Geometry check sheet. Reference: drawing and pictorial views, mm from the part's lowest x, y, z. Round coordinates to 2 decimals unless told otherwise and drop trailing zeros. Order: outer loops, then holes, each group sorted by start corner. A loop starts at its lowest first (then second) coordinate and runs counter-clockwise, first axis right, second up.
(1) Cross-section at B-B on z = 76.5. Enter the section's corners in (x, y), and give its area (3 significant figures).
(2) Cross-section at A-A on x = 61. Enter the section's corners in (y, z), and give its area (3 significant figures).
(3) Gauge pin test, flat ends, axial feed: P1, Ø1.4, axis at x = 37.5, y = 2, coming from the +Z side; P2, Ø1.5, axis at y = 1, z = 104.5, coming from the -X side (3 decimals); P3, Ø1.4, axis at x = 33, y = 1.5, coming from the -Z side. Record the tip position at first contact, or that the pin passes through.
(4) Thickness scan on L1, parallel to Z at x = 32.5, y = 2.15; L2, parallel to X at y = 0.2, z = 99; L3, parallel to Z at x = 62, y = 0.35. Record the ranges inside material, lowest first.
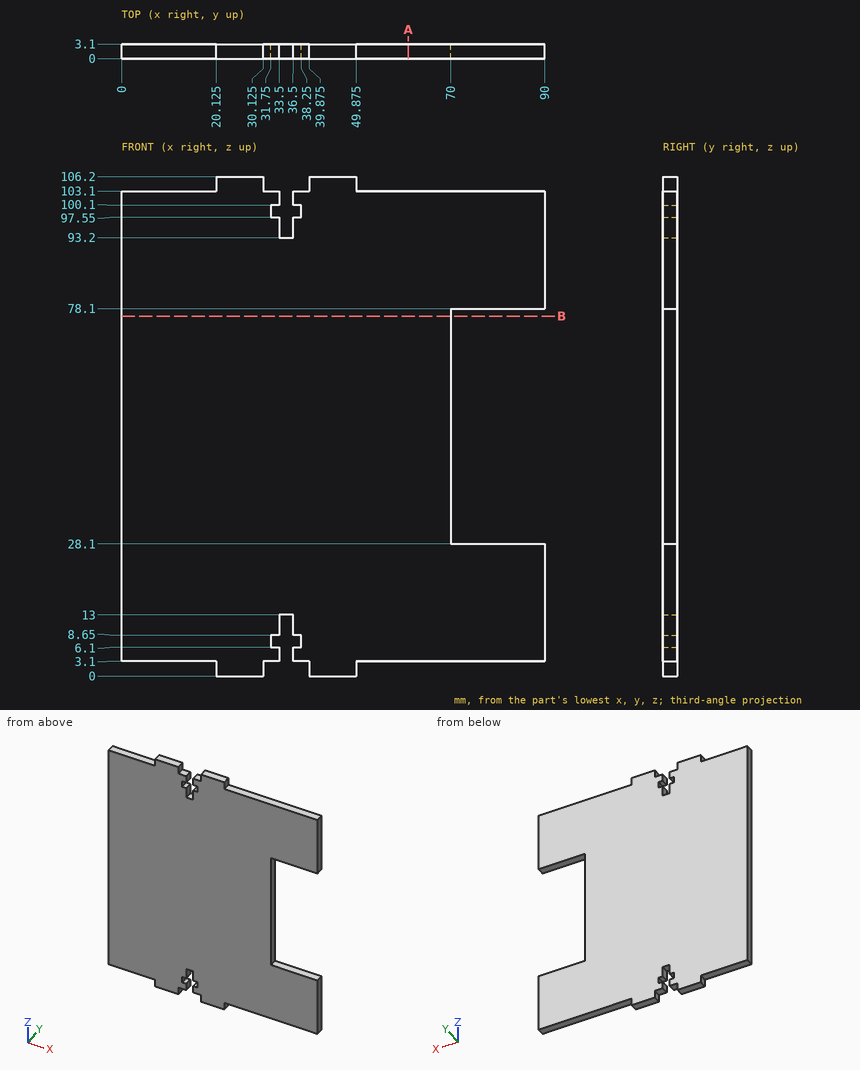
Found:
1. outline: (0, 0) - (70, 0) - (70, 3.1) - (0, 3.1) - close
1. area: 217 mm2
2. outline: (0, 3.1) - (3.1, 3.1) - (3.1, 103.1) - (0, 103.1) - close
2. area: 310 mm2
3. P1: stops at z = 103.1
3. P2: stops at x = 20.125
3. P3: stops at z = 3.1
4. L1: z = 3.1 to 6.1, 8.65 to 97.55, 100.1 to 103.1
4. L2: x = 0 to 31.75, 38.25 to 90
4. L3: z = 3.1 to 103.1
